Read the model definition and answer for the solid it produces. Units are mm, in the model's axes. Give positions to 0.01 mm unless a question says otherwise; leave off trailing zeros. Order: outer loops, then holes, each group sorted by start corner. A loop starts at its lowest first (then second) coordinate and runs counter-clockwise, first axis right, second up. Notation, with made-up numbers: (40.25, 35) -> (83.25, 35) arc R25 ccw to (83.25, 55) -> close; hole circle Ø10 at (-29, 73.25). An arc over 180 degrees is marked (long way). One line per question, with ' | ' between items. Start each with the question number.
```python
from build123d import *

# Parameters (mm, degrees)
F1_DEPTH = 22.606
F2_R     = 0.79375
F3_DEPTH = 19.0975001


with BuildPart() as f1:
    # F0 (on Top) → F1 (new body)
    with BuildSketch(Plane.XY):
        with BuildLine():
            ThreePointArc((-11.5859649124, 11.762037113), (0, 16.51), (11.5859649124, 11.762037113))
            Line((11.5859649124, 11.762037113), (12.7000000001, 12.8930022201))
            ThreePointArc((12.7000000001, 12.8930022201), (0, 18.0975), (-12.7000000001, 12.8930022201))
            Line((-12.7000000001, 12.8930022201), (-11.5859649124, 11.762037113))
        make_face()
    extrude(amount=F1_DEPTH)

    # F2 (on Front) → F3 (cut, up to face)
    with BuildSketch(Plane.XZ):
        with Locations((0, 11.303)):
            Circle(F2_R)
    extrude(amount=-F3_DEPTH, mode=Mode.SUBTRACT)


solid = f1.part
```
Q1. A cutting plane is placed at C-C, the plane z = 20.5. Determine the outline of the cut face in (x, y) (1 decimal).
Q2. A cutting plane is placed at A-A, the plane x = 0. Determine the outline of the cut face in (y, z), then the cut area to 3 significant figures.
Q3. A cutting plane is placed at D-D, the plane x = 10.5. Determine the outline of the cut face in (y, z).
Q4. Given P1, Ø3, axis at x = -8.5, y = 14, coming from the +Z side; P2, Ø1, axis at y = 16, z = 8.5, coming from the -X side; P3, Ø2, axis at x = -4, z = 19.5, coming from the +Y side; P4, Ø1.4, axis at x = 0, z = 11.303, coming from the +Y side, each flat-ended and moving along its own axis, determine where each tip first touches the part or whether it passes through.
Q5. A cutting plane is placed at B-B, the plane y = 14. Determine the outline of the cut face in (x, z), then the cut area to 3 significant figures.
Q6. Find the intervals of material crossed by line 1 (Z direction, x = 0, y = 17.15); line 2 (X direction, y = 13.5, z = 19.75); line 3 (X direction, y = 14.75, z = 7.75), in increasing order.
Geometry results:
1) outline: (-12.7, 12.9) -> (-11.6, 11.8) arc R16.5 cw to (11.6, 11.8) -> (12.7, 12.9) arc R18.1 ccw to start
2) outline: (16.51, 0) -> (18.1, 0) -> (18.1, 10.51) -> (16.51, 10.51) -> close; (16.51, 12.1) -> (18.1, 12.1) -> (18.1, 22.61) -> (16.51, 22.61) -> close | area: 33.4 mm²
3) outline: (12.74, 0) -> (14.74, 0) -> (14.74, 22.61) -> (12.74, 22.61) -> close
4) P1: z = 22.61 | P2: x = -9.34 | P3: y = 17.85 | P4: through
5) outline: (-11.47, 0) -> (-8.75, 0) -> (-8.75, 22.61) -> (-11.47, 22.61) -> close; (8.75, 0) -> (11.47, 0) -> (11.47, 22.61) -> (8.75, 22.61) -> close | area: 123 mm²
6) line 1: 0 to 10.51, 12.1 to 22.61 | line 2: -12.05 to -9.5, 9.5 to 12.05 | line 3: -10.49 to -7.42, 7.42 to 10.49
